Part model, mm, in its own coordinate system. A direction names the side the tool comes from. Round coordinates to 2 decimals unless told otherwise and drop trailing zeros. Write each loop counter-clockwise with the first axis right and the second up, starting at its lowest first coordinate (ties: lowest second). Pieces come first, ordered by that corner, then holes.
```python
from build123d import *

# Parameters (mm, degrees)
F0_W     = 6.35
F0_H     = 254
F1_DEPTH = 279.4
F3_DEPTH = 25.4
F4_W     = 79.375
F4_H     = 12.7
F5_DEPTH = 25.4
F7_D     = 6.35


with BuildPart() as f1:
    # F0 (on Front) → F1 (new body)
    with BuildSketch(Plane.XZ):
        Rectangle(F0_W, F0_H)
    extrude(amount=F1_DEPTH)

    # F2 (on face) → F3 (cut)
    with BuildSketch(Plane(origin=(-3.175, 0, 0), x_dir=(0, -1, 0), z_dir=(-1, 0, 0))):
        with BuildLine():
            Line((0, 82.671984), (16.538269, 82.671984))
            Line((16.538269, 82.671984), (174.625, 47.625))
            Line((174.625, 47.625), (12.7, 47.625))
            ThreePointArc((12.7, 47.625), (60.126734, -66.873266), (174.625, -114.3))
            Line((174.625, -114.3), (279.4, -114.3))
            Line((279.4, -114.3), (279.4, 127))
            Line((279.4, 127), (0, 127))
            Line((0, 127), (0, 82.671984))
        make_face()
        with BuildLine():
            Line((174.625, 47.625), (16.538269, 82.671984))
            ThreePointArc((16.538269, 82.671984), (13.662427, 65.253269), (12.7, 47.625))
            Line((12.7, 47.625), (174.625, 47.625))
        make_face()
    extrude(amount=-F3_DEPTH, mode=Mode.SUBTRACT)

    # F4 (on face) → F5 (cut)
    with BuildSketch(Plane(origin=(-3.175, 0, 0), x_dir=(0, -1, 0), z_dir=(-1, 0, 0))):
        with Locations((239.7125, -120.65)):
            Rectangle(F4_W, F4_H)
    extrude(amount=-F5_DEPTH, mode=Mode.SUBTRACT)

    # F7 (through all)
    with Locations(Plane.YZ.offset(3.175)):
        with Locations((-187.325, -120.65), (-101.6, -114.3), (-41.275, -68.652838), (-9.525, -2.670206), (-8.269135, 69.937184)):
            Hole(F7_D / 2)


solid = f1.part
```
Q1. Cut at A-A on z = -120.65. Write the cut outline in (x, y) (3 decimals).
Values follow:
outline: (-3.175, -200.025) - (3.175, -200.025) - (3.175, -190.5) - (-3.175, -190.5) - close; (-3.175, -184.15) - (3.175, -184.15) - (3.175, 0) - (-3.175, 0) - close
Q2. Cut at C-C on x = 1. Write the cut outline in (y, z) (3 decimals), plus the area to 3 significant figures.
Values follow:
outline: (-200.025, -127) - (0, -127) - (0, 82.672) - (-16.538, 82.672) arc R161.925 cw to (-12.7, 47.625) arc R161.925 cw to (-174.625, -114.3) - (-200.025, -114.3) - close; hole circle Ø6.35 at (-187.325, -120.65); hole circle Ø6.35 at (-101.6, -114.3); hole circle Ø6.35 at (-41.275, -68.653); hole circle Ø6.35 at (-9.525, -2.67); hole circle Ø6.35 at (-8.269, 69.937)
area: 10,600 mm2
Q3. Cut at D-D on y = -122. Write the cut outline in (x, z) (3 decimals).
Values follow:
outline: (-3.175, -127) - (3.175, -127) - (3.175, -105.51) - (-3.175, -105.51) - close
Q4. Cut at B-B on y = -101.6. Write the cut outline in (x, z) (3 decimals), plus the area to 3 significant figures.
Values follow:
outline: (-3.175, -127) - (3.175, -127) - (3.175, -117.475) - (-3.175, -117.475) - close; (-3.175, -111.125) - (3.175, -111.125) - (3.175, -96.899) - (-3.175, -96.899) - close
area: 151 mm2
Q5. Wall check: L1, parallel to Y at x = -0.75, z = -3; L2, parallel to Z at x = -1.25, y = -41; L3, parallel to Z at x = 0.25, y = -185. Give the ranges that are in metal, low to high.
Values follow:
L1: y = -20.82 to -12.68, -6.37 to 0
L2: z = -127 to -71.82, -65.49 to -43.83
L3: z = -127 to -122.81, -118.49 to -114.3
Q6. Mould opens along Y. For faces 4 (the cylindrical face through (-0.044, -12.553, -1.717)), 5 (the cylindrical face through (-0.044, -58.875, -65.607)), 6 (the flat face through (3.175, -55, -77)), 7 (the flat face through (0, 0, -21)) say: +Y half, -Y half, draft (parallel to the pull), parting line (faces both ways), or undercut.
Values follow:
face 4: undercut
face 5: -Y half
face 6: draft
face 7: +Y half
Q7. Drop flat-ended pins along their axis: pin 1 (5 mm diameter, centred on y = -101.6, z = -114.3, fed in from -X); pin 2 (3 mm diameter, centred on x = 0, y = -184.5, fed in from +Z). Give the stop position or say it passes through.
Values follow:
pin 1: passes through
pin 2: stops at z = -114.3
Q8. Which spindle directions (+Z, -Z, +X, -X, +Y, -Y) get a long thin tool onto all of the face, cutting with end or side? Do faces 1 (the flat face through (0, -187, -114.3)), 2 (the cylindrical face through (-0.04, -186.64, -123.75)), 3 (the cylindrical face through (-0.04, -13.69, 65.5)). Say none if no direction does.
Values follow:
face 1: +Z, +X, -X, -Y
face 2: +X, -X
face 3: +X, -X, -Y
